Read the model definition and answer for the solid it produces. Units are mm, in the model's axes. A direction names the side the tool comes from. Coordinates: 2 decimals unless noted, no trailing zeros. Write each loop counter-clockwise with the first axis right and the second up, starting at its lowest first coordinate (ties: lowest second). Pieces come first, ordered by that corner, then holes.
1) Each of these flat-tipped pins is pushed along its axis until it touches: pin 1 Ø9.5 at (y, z) = (36.5, 11.5) entering from +X; pin 2 Ø11 at (x, z) = (-26.5, 22.5) entering from +Y; pin 3 Ø16 at (x, z) = (27.5, 21) entering from +Y; pin 4 Ø8.5 at (x, z) = (-26.86, 15.88) entering from +Y. Where does it stop, or does it pass through?
2) The part is cut by section A-A (z = 19.5). Determine the outline of the cut face in (x, y) (3 decimals), then the cut area to 3 significant figures.
3) Find the intervals of material crossed by line 1 (Y direction, x = -19, z = 22); line 2 (X direction, y = 37, z = 6); line 3 (X direction, y = 13.5, z = 3), in increasing order.
4) The part is cut by section B-B (z = 5.5). Determine the outline of the cut face in (x, y) (3 decimals), then the cut area to 3 significant figures.
5) Determine the mould class of faces 1 (the face through (28, 0, 16)), 2 (the face through (-21.466, -0.619, 15.638)), 3 (the face through (-11.618, -15, 16)) for opening direction X: +X half, -X half, draft (parallel to the pull), parting line (faces both ways), or undercut.
6) The part is cut by section C-C (x = -19). Determine the outline of the cut face in (y, z), then the cut area to 3 significant figures.
7) The part is cut by section D-D (y = 26.5). Determine the outline of the cut face in (x, z), then the cut area to 3 significant figures.
8) Which of the six approach directions +Z, -Z, +X, -X, +Y, -Y give full straight-line access (tool end or side, diameter ignored) to faces 4 (the face through (-32, 4.854, 19)), 5 (the face through (-22, -5.941, 19)), 6 (the face through (-38.161, -1, 16)), 7 (the face through (0, 29, 16))?
from build123d import *

# Parameters (mm, degrees)
BOSS_EXTRUDE1_DEPTH          = 31.75
F_3_8_0_375_DIAMETER_HOLE1_D = 10.795
FILLET1_R                    = 1.27
FILLET2_R                    = 6.35


with BuildPart() as part:
    # Sketch1 → Boss-Extrude1 (new body)
    with BuildSketch(Plane.XY):
        Polygon((0, 0), (50.8, 0), (50.8, -9.525), (-3.3628076, -23.086314), (-11.6178076, -23.086314), (-11.6178076, -5.941314), (-38.1608076, -5.941314), (-38.1608076, 4.853686), (-15.3008076, 4.853686), (-6.35, 50.8), (0, 50.8), align=None)
    extrude(amount=BOSS_EXTRUDE1_DEPTH)

    # 3/8 (0.375) Diameter Hole1 (through all)
    with Locations(Plane(origin=(0, 4.853686, 0), x_dir=(1, 0, 0), z_dir=(0, 1, 0))):
        with Locations((-26.8578076, -15.875)):
            Hole(F_3_8_0_375_DIAMETER_HOLE1_D / 2)

    # Fillet1
    fillet1_edges = [part.edges().sort_by_distance(p)[0] for p in [
        (-15.3008076, 4.853686, 15.875),
    ]]
    fillet(fillet1_edges, radius=FILLET1_R)

    # Fillet2
    fillet2_edges = [part.edges().sort_by_distance(p)[0] for p in [
        (0, 0, 15.875),
    ]]
    fillet(fillet2_edges, radius=FILLET2_R)


solid = part.part
Reported:
1. pin 1: stops at x = 0
1. pin 2: stops at y = 4.85
1. pin 3: stops at y = 0
1. pin 4: passes through
2. outline: (-38.161, -5.941) - (-30.857, -5.941) - (-30.857, 4.854) - (-38.161, 4.854) - close; (-22.859, -5.941) - (-11.618, -5.941) - (-11.618, -23.086) - (-3.363, -23.086) - (50.8, -9.525) - (50.8, 0) - (6.35, 0) arc R6.35 cw to (0, 6.35) - (0, 50.8) - (-6.35, 50.8) - (-15.101, 5.881) arc R1.27 cw to (-16.347, 4.854) - (-22.859, 4.854) - close
2. area: 1,840 mm2
3. line 1: y = -5.94 to 4.85
3. line 2: x = -9.04 to 0
3. line 3: x = -13.62 to 0
4. outline: (-38.161, -5.941) - (-11.618, -5.941) - (-11.618, -23.086) - (-3.363, -23.086) - (50.8, -9.525) - (50.8, 0) - (6.35, 0) arc R6.35 cw to (0, 6.35) - (0, 50.8) - (-6.35, 50.8) - (-15.101, 5.881) arc R1.27 cw to (-16.347, 4.854) - (-38.161, 4.854) - close
4. area: 1,920 mm2
5. face 1: draft
5. face 2: undercut
5. face 3: -X half
6. outline: (-5.94, 0) - (4.85, 0) - (4.85, 31.75) - (-5.94, 31.75) - close
6. area: 343 mm2
7. outline: (-11.08, 0) - (0, 0) - (0, 31.75) - (-11.08, 31.75) - close
7. area: 352 mm2
8. face 4: +Z, -Z, -X, +Y
8. face 5: +Z, -Z, -X, -Y
8. face 6: +Z, -Z, -X, +Y, -Y
8. face 7: +Z, -Z, +X, +Y
